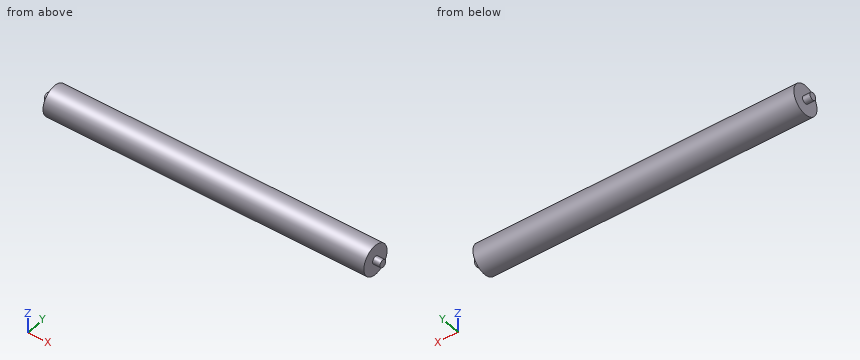
```python
from build123d import *

# Parameters (mm, degrees)
F0_R     = 9.525
F1_DEPTH = 19.05
F2_R     = 38.1
F3_DEPTH = 825.5
F4_R     = 9.525
F5_DEPTH = 19.05


with BuildPart() as f1:
    # F0 (on Right) → F1 (new body)
    with BuildSketch(Plane.YZ):
        Circle(F0_R)
    extrude(amount=-F1_DEPTH)

    # F2 (on face) → F3 (join)
    with BuildSketch(Plane(origin=(-19.05, 0, 0), x_dir=(0, -1, 0), z_dir=(-1, 0, 0))):
        Circle(F2_R)
    extrude(amount=F3_DEPTH)

    # F4 (on face) → F5 (join)
    with BuildSketch(Plane(origin=(-844.55, 0, 0), x_dir=(0, -1, 0), z_dir=(-1, 0, 0))):
        Circle(F4_R)
    extrude(amount=F5_DEPTH)


solid = f1.part
```
Input: part model. Units: mm. Frame: model coordinates. Give positions to 0.01 mm unless a question says otherwise; leave off trailing zeros. Write each loop counter-clockwise with the first axis right and the second up, starting at its lowest first coordinate (ties: lowest second). Pieces come first, ordered by that corner, then holes. Notation, with made-up numbers: (81, 42) - (123, 42) arc R32 ccw to (123, 72) - close; hole circle Ø5 at (58.25, -0.75). An arc over 180 degrees is marked (long way). Write item = value, one per line. Start each with the question number.
1) Material intervals for L1, parallel to X at y = 7.5, z = -19; L2, parallel to Y at x = -61, z = 3.5; L3, parallel to Y at x = -738.5, z = 10, sorted ascending. Write a range as [from, to].
2) Cut plane A-A (y = 0). Return loops of the section in (x, z) (3 decimals).
3) Cut plane C-C (x = -752.5). Return loops of the section in (y, z).
4) Pin query (flat end, axial travel): pin 1 (10 mm diameter, centred on x = -146.5, z = -15, fed in from -Y); pin 2 (2 mm diameter, centred on x = -608, z = -21.5, fed in from -Y); pin 3 (12 mm diameter, centred on y = -20.5, z = -14.5, fed in from -X). Return the tip coordinate at first contact, or that it passes through.
Answers follow:
q1.L1 = [-844.55, -19.05]
q1.L2 = [-37.94, 37.94]
q1.L3 = [-36.76, 36.76]
q2.outline = (-863.6, -9.525) - (-844.55, -9.525) - (-844.55, -38.1) - (-19.05, -38.1) - (-19.05, -9.525) - (0, -9.525) - (0, 9.525) - (-19.05, 9.525) - (-19.05, 38.1) - (-844.55, 38.1) - (-844.55, 9.525) - (-863.6, 9.525) - close
q3.outline = circle Ø76.2 at (0, 0)
q4.pin_1 = -36.76
q4.pin_2 = -32.11
q4.pin_3 = -844.55
